from build123d import *

# Parameters (mm, degrees)
SKETCH1_W                  = 50
SKETCH1_H                  = 173.07
BOSS_EXTRUDE1_DEPTH        = 5.2
CUT_EXTRUDE1_DEPTH         = 6
SKETCH4_W                  = 5.2
SKETCH4_H                  = 5.7
CUT_EXTRUDE2_DEPTH         = 6
CHAMFER1_SIZE              = 3
LPATTERN1_COUNT            = 11
LPATTERN1_PITCH            = 15
CHAMFER1_OF_LPATTERN1_SIZE = 3


with BuildPart() as part:
    # Sketch1 → Boss-Extrude1 (new body)
    with BuildSketch(Plane(origin=(0, 0, 0), x_dir=(1, 0, 0), z_dir=(0, 1, 0))):
        with Locations((25, 86.535)):
            Rectangle(SKETCH1_W, SKETCH1_H)
    extrude(amount=BOSS_EXTRUDE1_DEPTH)

    # Sketch2 → Cut-Extrude1 (cut)
    with BuildSketch(Plane(origin=(0, 5.2, 0), x_dir=(1, 0, 0), z_dir=(0, 1, 0))):
        Polygon((0, 134.785728753), (14.142135624, 148.927864376), (0, 163.07), align=None)
        Polygon((14.142135624, 20.927864376), (0, 6.785728753), (0, 35.07), align=None)
    extrude(amount=-CUT_EXTRUDE1_DEPTH, mode=Mode.SUBTRACT)

    # Sketch4 → Cut-Extrude2 (cut)
    with BuildSketch(Plane(origin=(0, 5.2, 0), x_dir=(1, 0, 0), z_dir=(0, 1, 0))):
        with Locations((47.4, 160.22)):
            Rectangle(SKETCH4_W, SKETCH4_H)
    cut_extrude2 = extrude(amount=-CUT_EXTRUDE2_DEPTH, mode=Mode.SUBTRACT)

    # Chamfer1
    chamfer1_edges = [part.edges().sort_by_distance(p)[0] for p in [
        (50, 2.6, -163.07),
        (50, 2.6, -157.37),
    ]]
    chamfer(chamfer1_edges, length=CHAMFER1_SIZE)

    # LPattern1: Cut-Extrude2 ×11
    with Locations(*[(0, 0, i * LPATTERN1_PITCH) for i in range(1, LPATTERN1_COUNT)]):
        add(cut_extrude2, mode=Mode.SUBTRACT)

    # Chamfer1 of LPattern1
    chamfer1_of_lpattern1_edges = [part.edges().sort_by_distance(p)[0] for p in [
        (50, 2.6, -148.07),
        (50, 2.6, -142.37),
        (50, 2.6, -133.07),
        (50, 2.6, -127.37),
        (50, 2.6, -118.07),
        (50, 2.6, -112.37),
        (50, 2.6, -103.07),
        (50, 2.6, -97.37),
        (50, 2.6, -88.07),
        (50, 2.6, -82.37),
        (50, 2.6, -73.07),
        (50, 2.6, -67.37),
        (50, 2.6, -58.07),
        (50, 2.6, -52.37),
        (50, 2.6, -43.07),
        (50, 2.6, -37.37),
        (50, 2.6, -28.07),
        (50, 2.6, -22.37),
        (50, 2.6, -13.07),
        (50, 2.6, -7.37),
    ]]
    chamfer(chamfer1_of_lpattern1_edges, length=CHAMFER1_OF_LPATTERN1_SIZE)


solid = part.part
Here's how the part is built. I have some questions about the finished solid (model axes, mm). A direction names the side the tool comes from. Round coordinates to 2 decimals unless told otherwise and drop trailing zeros. Write each loop counter-clockwise with the first axis right and the second up, starting at its lowest first coordinate (ties: lowest second). Pieces come first, ordered by that corner, then holes.
1. For faces 4 (the flat face through (0, 3, -3)), 5 (the flat face through (6.97, 2.64, -28.1)), 6 (the flat face through (48.52, 2.64, -20.85)), which set-ups out of +Z, -Z, +X, -X, +Y, -Y let a thin tool reach every point of the face, with its end or its side?
2. Suppose I cut it at B-B (z = -54.5). List the corners of the cut face in (x, y) for me.
3. If we mould it in two halves opening along Z, with no side actions, what happens to faces 1 (the flat face through (48.52, 2.64, -110.85)), 2 (the flat face through (25, 3, 0)), 3 (the flat face through (50, 3, -123))? For each: released by +Z, released by -Z, zero draft, split by the parting line, or undercut.
4. Suppose I cut it at A-A (x = 4). List the corners of the cut face in (y, z) for me.
5. I need wall thicknesses on L1, parallel to Z at x = 4, y = 1.8; L2, parallel to Z at x = 8, y = 0.45; L3, parallel to X at y = 2.2, z = -12. Which ranges of each line are inside material? Lowest first, please.
6. Will these pins go through, and if not, where does the flat tip stop? pin 1 Ø1.6 at (y, z) = (1.5, -114.5) entering from +X; pin 2 Ø3 at (x, z) = (15, -124.5) entering from -Y.
Answer sheet:
1. face 4: +Z, -Z, -X, +Y, -Y
1. face 5: -X, +Y, -Y
1. face 6: +X, +Y, -Y
2. outline: (0, 0) - (44.8, 0) - (44.8, 5.2) - (0, 5.2) - close
3. face 1: undercut
3. face 2: released by +Z
3. face 3: zero draft
4. outline: (0, -173.07) - (5.2, -173.07) - (5.2, -159.07) - (0, -159.07) - close; (0, -138.79) - (5.2, -138.79) - (5.2, -31.07) - (0, -31.07) - close; (0, -10.79) - (5.2, -10.79) - (5.2, 0) - (0, 0) - close
5. L1: z = -173.07 to -159.07, -138.79 to -31.07, -10.79 to 0
5. L2: z = -173.07 to -155.07, -142.79 to -27.07, -14.79 to 0
5. L3: x = 5.21 to 44.8
6. pin 1: stops at x = 44.8
6. pin 2: stops at y = 0
